```python
from build123d import *

# Parameters (mm, degrees)
SKETCH1_R           = 15
BOSS_EXTRUDE1_DEPTH = 8
SKETCH2_R           = 5
BOSS_EXTRUDE2_DEPTH = 1
SKETCH3_R           = 3
BOSS_EXTRUDE3_DEPTH = 9.5
HOLE1_D             = 4
HOLE1_CBORE_D       = 8
HOLE1_CBORE_DEPTH   = 5


with BuildPart() as part:
    # Sketch1 → Boss-Extrude1 (new body)
    with BuildSketch(Plane(origin=(0, 0, 0), x_dir=(1, 0, 0), z_dir=(0, 1, 0))):
        Circle(SKETCH1_R)
    extrude(amount=BOSS_EXTRUDE1_DEPTH)

    # Sketch2 → Boss-Extrude2 (add)
    with BuildSketch(Plane(origin=(0, 8, 0), x_dir=(1, 0, 0), z_dir=(0, 1, 0))):
        Circle(SKETCH2_R)
    extrude(amount=BOSS_EXTRUDE2_DEPTH)

    # Sketch3 → Boss-Extrude3 (add)
    with BuildSketch(Plane(origin=(0, 9, 0), x_dir=(1, 0, 0), z_dir=(0, 1, 0))):
        Circle(SKETCH3_R)
    extrude(amount=BOSS_EXTRUDE3_DEPTH)

    # Hole1 (through all)
    with Locations(Plane(origin=(0, 8, 0), x_dir=(1, 0, 0), z_dir=(0, 1, 0))):
        with Locations((-10, 0), (0, 10), (10, 0), (0, -10)):
            CounterBoreHole(HOLE1_D / 2, HOLE1_CBORE_D / 2, HOLE1_CBORE_DEPTH)


solid = part.part
```
Could you check a few things on this model? Use its own coordinates, in mm. A direction names the side the tool comes from. Coordinates: 2 decimals unless noted, no trailing zeros. Loops run counter-clockwise (first coordinate to the right, second up) from the corner with the lowest first, then second, coordinate; pieces in that order, holes last.
1) Please list where these lines run through material, in increasing order: line 1 along Z through (x, y) = (0, 2.4); line 2 along Z through (x, y) = (0, 6.6); line 3 along X through (y, z) = (4.5, 1).
Reported:
line 1: z = -15 to -12, -8 to 8, 12 to 15
line 2: z = -15 to -14, -6 to 6, 14 to 15
line 3: x = -14.97 to -13.87, -6.13 to 6.13, 13.87 to 14.97
2) Imagine slicing it at A-A (x = 0). List the corners of the cut face in (y, z) for me, and give its area (3 significant figures).
Reported:
outline: (0, -15) - (8, -15) - (8, -14) - (3, -14) - (3, -12) - (0, -12) - close; (0, -8) - (3, -8) - (3, -6) - (8, -6) - (8, -5) - (9, -5) - (9, -3) - (18.5, -3) - (18.5, 3) - (9, 3) - (9, 5) - (8, 5) - (8, 6) - (3, 6) - (3, 8) - (0, 8) - close; (0, 12) - (3, 12) - (3, 14) - (8, 14) - (8, 15) - (0, 15) - close
area: 203 mm2
3) Imagine slicing it at B-B (z = 0). List the corners of the cut face in (x, y) for me.
Reported:
outline: (-15, 0) - (-12, 0) - (-12, 3) - (-14, 3) - (-14, 8) - (-15, 8) - close; (-8, 0) - (8, 0) - (8, 3) - (6, 3) - (6, 8) - (5, 8) - (5, 9) - (3, 9) - (3, 18.5) - (-3, 18.5) - (-3, 9) - (-5, 9) - (-5, 8) - (-6, 8) - (-6, 3) - (-8, 3) - close; (12, 0) - (15, 0) - (15, 8) - (14, 8) - (14, 3) - (12, 3) - close
4) Imagine slicing it at C-C (y = 5). List the corners of the cut face in (x, z) for me.
Reported:
outline: circle Ø30 at (0, 0); hole circle Ø8 at (-10, 0); hole circle Ø8 at (0, -10); hole circle Ø8 at (0, 10); hole circle Ø8 at (10, 0)
5) Thinking about a two-plate mould opening in X: for faces 1 (the face through (0, 1, 8)), 2 (the face through (-0.1, 9, 3.3)), 3 (the face through (-1.08, 8.49, 4.88)), which applies, released by +X, released by -X, zero draft, split by the parting line, or undercut?
Reported:
face 1: undercut
face 2: zero draft
face 3: split by the parting line
6) Imagine slicing it at D-D (x = 10). List the corners of the cut face in (y, z) for me.
Reported:
outline: (0, -11.18) - (8, -11.18) - (8, -4) - (3, -4) - (3, -2) - (0, -2) - close; (0, 2) - (3, 2) - (3, 4) - (8, 4) - (8, 11.18) - (0, 11.18) - close
7) Will these pins go through, and if not, where does the flat tip stop? pin 1 Ø4 at (x, z) = (-11.5, 0) entering from +Y; pin 2 Ø4 at (y, z) = (2.5, 9) entering from -X; pin 3 Ø13 at (x, z) = (0, 10) entering from +Y.
Reported:
pin 1: stops at y = 3
pin 2: stops at x = -13.27
pin 3: stops at y = 9
8) Which directions (+Z, -Z, +X, -X, +Y, -Y) give clear straight access to the entire face, cutting with the end or side of a thin tool? Please do faces 4 (the face through (-13.2, 5.5, 2.4)), 5 (the face through (-8.4, 1.5, 1.2)).
Reported:
face 4: +Y
face 5: +Y, -Y
